```python
from build123d import *

# Parameters (mm, degrees)
SKETCH1_R                = 4
SKETCH1_R_2              = 1.4
BOSS_EXTRUDE1_DEPTH      = 8
OUTSIDE_CURVES_R         = 5
INSIDE_CURVES_R          = 3
BOLT_HOLES_DEPTH         = 3
SKETCH3_R                = 1.4
BEARING_SCREW_HOLE_DEPTH = 10
SKETCH5_R                = 6
BEARINGS_DEPTH           = 8.5
SKETCH6_R                = 2.75
SCREW_DEPTH              = 3.5


with BuildPart() as part:
    # Sketch1 → Boss-Extrude1 (new body)
    with BuildSketch(Plane.XY):
        Polygon((-11, -3), (-11, -10), (-40, -10), (-40, 10), (40, 10), (40, -10), (11, -10), (11, -3), align=None)
        with Locations((-30, 0)):
            Circle(SKETCH1_R, mode=Mode.SUBTRACT)
        with Locations((-20, 4)):
            Circle(SKETCH1_R_2, mode=Mode.SUBTRACT)
        with Locations(Location((20, 4, 0), (0, 0, 180))):
            Circle(SKETCH1_R_2, mode=Mode.SUBTRACT)
        with Locations(Location((30, 0, 0), (0, 0, 180))):
            Circle(SKETCH1_R, mode=Mode.SUBTRACT)
    extrude(amount=BOSS_EXTRUDE1_DEPTH)

    # outside curves
    outside_curves_edges = [part.edges().sort_by_distance(p)[0] for p in [
        (-40, -10, 4),
        (-40, 10, 4),
        (40, 10, 4),
        (40, -10, 4),
    ]]
    fillet(outside_curves_edges, radius=OUTSIDE_CURVES_R)

    # inside curves
    inside_curves_edges = [part.edges().sort_by_distance(p)[0] for p in [
        (-11, -10, 4),
        (11, -10, 4),
    ]]
    fillet(inside_curves_edges, radius=INSIDE_CURVES_R)

    # Sketch2 → bolt holes (cut)
    with BuildSketch(Plane.XY.offset(8)):
        Polygon((-17, 4), (-18.5, 6.598076211), (-21.5, 6.598076211), (-23, 4), (-21.5, 1.401923789), (-18.5, 1.401923789), align=None)
        Polygon((18.5, 1.401923789), (17, 4), (18.5, 6.598076211), (21.5, 6.598076211), (23, 4), (21.5, 1.401923789), align=None)
    extrude(amount=-BOLT_HOLES_DEPTH, mode=Mode.SUBTRACT)

    # Sketch3 → bearing screw hole (cut)
    with BuildSketch(Plane.XZ.offset(3)):
        with Locations(Location((0, 4, 0), (0, 0, 270))):
            Circle(SKETCH3_R)
    extrude(amount=-BEARING_SCREW_HOLE_DEPTH, mode=Mode.SUBTRACT)

    # Sketch5 → bearings (add)
    with BuildSketch(Plane.XZ.offset(3)):
        with Locations(Location((0, 4, 0), (0, 0, 41.810314896))):
            Circle(SKETCH5_R)
    extrude(amount=BEARINGS_DEPTH)

    # Sketch6 → screw (add)
    with BuildSketch(Plane.XZ.offset(11.5)):
        with Locations(Location((0, 4, 0), (0, 0, 270))):
            Circle(SKETCH6_R)
    extrude(amount=SCREW_DEPTH)


solid = part.part
```
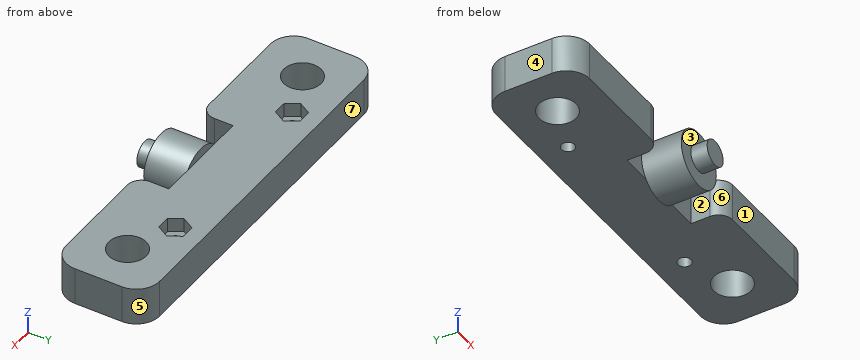
Geometry check sheet. Reference: the model listing, model coordinates, mm. Face numbers are marked on the shaded views. A direction names the side the tool comes from. Coordinates: 2 decimals unless noted, no trailing zeros. Write each loop counter-clockwise with the first axis right and the second up, starting at its lowest first coordinate (ties: lowest second). Pieces come first, ordered by that corner, then holes. Notation, with made-up numbers: M -16.5,-10 L 4.5,-10 A29 cw 4.5,26 Z; hole C -3,76.25 d5. An arc over 180 degrees is marked long. One line per item, written item: value. Start each with the question number.
(1) Sectioned sample at A-A, the plane y = 0. Enter the section's corners in (x, z).
(2) Depth check by flat-ended pin: pin 1 (12 mm diameter, centred on x = 17, y = -0.5, fed in from +Z); pin 2 (13 mm diameter, centred on x = -30, y = 0, fed in from -Z); pin 3 (3.5 mm diameter, centred on x = -19.5, z = 7, fed in from -Y). Enter the tip coordinate at first touch or a pass-through.
(3) Tool access check on the marked faces 1, 2 and 3. Record the directions out of +Z, -Z, +X, -X, +Y, -Y that give a thin tool (end or side, any length) a straight path to the whole face; none if there is none.
(4) Scan lines: line 1 along Y through (x, z) = (-20, 3.2); line 2 along X through (y, z) = (-2, 3.5); line 3 along X through (y, z) = (-6.75, 4.5). Record each from-to range of solid material in increasing order. Write a range as [from, to].
(5) Sectioned sample at D-D, the plane x = 27. Enter the section's corners in (y, z).
(6) Release check for a two-part mould opening along X. For the marked faces 4, 5, 6 and 7 record: released by +X, released by -X, zero draft, split by the parting line, or undercut.
(7) Sectioned sample at C-C, the plane z = 4. State how many separate pieces and enclosed holes the cut face has, and give its area (3 significant figures).
(8) Sectioned sample at B-B, the plane x = 0. Enter the section's corners in (y, z).
Filled sheet:
1. outline: M -40,0 L -34,0 L -34,8 L -40,8 Z; M -26,0 L 26,0 L 26,8 L -26,8 Z; M 34,0 L 40,0 L 40,8 L 34,8 Z; hole C 0,4 d2.8
2. pin 1: z = 8
2. pin 2: z = 0
2. pin 3: y = -10
3. face 1: +Z, -Z, +X, -Y
3. face 2: +Z, -Z, -Y
3. face 3: -Y
4. line 1: [-10, 2.6], [5.4, 10]
4. line 2: [-40, -33.46], [-26.54, -1.31], [1.31, 26.54], [33.46, 40]
4. line 3: [-39.68, -11], [-5.98, 5.98], [11, 39.68]
5. outline: M -10,0 L -2.65,0 L -2.65,8 L -10,8 Z; M 2.65,0 L 10,0 L 10,8 L 2.65,8 Z
6. face 4: released by -X
6. face 5: released by +X
6. face 6: undercut
6. face 7: zero draft
7. separate pieces: 1
7. enclosed holes: 5
7. area: 1,400 mm²
8. outline: M -15,1.25 L -11.5,1.25 L -11.5,-2 L -3,-2 L -3,0 L 10,0 L 10,8 L -3,8 L -3,10 L -11.5,10 L -11.5,6.75 L -15,6.75 Z; hole M -3,2.6 L 7,2.6 L 7,5.4 L -3,5.4 Z
